Geometry: final body of the model. Coordinates: model frame, mm. A direction names the side the tool comes from. Round coordinates to 2 decimals unless told otherwise and drop trailing zeros. Write each loop counter-clockwise with the first axis right and the second up, starting at its lowest first coordinate (ties: lowest second). Pieces come first, ordered by that corner, then holes. Notation, with made-up numbers: M 86.25,74 L 110.25,74 A27 ccw 110.25,95 Z; hole C 79.25,18.25 d10. An arc over 180 degrees is marked long. Answer as CSV lines item,"result". Start each with the question number.
Q1. Section query A-A on y = 112.5. Output: boundary loops of the cut face in (x, z).
Q2. Section query C-C on x = 33. Output: boundary loops of the cut face in (y, z), and give its area (3 significant figures).
Q3. Section query B-B on z = 12.5. Output: boundary loops of the cut face in (x, y) (3 decimals), and give its area (3 significant figures).
Q4. First-contact query: pin 1 (4 mm diameter, centred on x = 86.5, y = 33, fed in from -Z); pin 2 (6 mm diameter, centred on y = 212.775, z = 4.5, fed in from +X); pin 3 (4.5 mm diameter, centred on x = 85, y = 132.5, fed in from -Z). Flat tips, straight axial feed; report the tip coordinate or a pass-through.
Q5. Ray query, probe 1 along X at (y, z) = (42.5, 14.5); probe 2 along X at (y, z) = (77.5, 14.25); probe 3 along Y at (x, z) = (-73.75, 4.5) (3 decimals). Return the intervals inside material, ascending.
Q6. Reachability of faces 4 (the flat face through (-87.9, 34.3, 2.1)), 5 (the flat face through (82, 137.775, 10)), 6 (the flat face through (-61.6, 30.1, 4.9)) from +Z, -Z, +X, -X, +Y, -Y: full face, straight path, thin tool, end or side. Return the list, or none.
Q7. Mould query, pull axis X, two halves, no side actions, for faces 1 (the flat face through (-81.5, 112, 15)), 2 (the flat face through (-82.5, 214, 7)), 3 (the flat face through (87, 133, 9)). Classes: pulls with the +X half, pulls with the -X half, needs draft (parallel to the pull), parting line crosses it, or undercut.
Q8. Section query D-D on y = 181.5. Output: boundary loops of the cut face in (x, z).
```python
from build123d import *

# Parameters (mm, degrees)
BOSS_EXTRUDE1_DEPTH = 10
BOSS_EXTRUDE2_DEPTH = 10
SKETCH3_W           = 9
SKETCH3_H           = 9
CUT_EXTRUDE2_DEPTH  = 10
SKETCH5_W           = 9
SKETCH5_H           = 9
CUT_EXTRUDE3_DEPTH  = 10
SKETCH6_R           = 2.25
CUT_EXTRUDE4_DEPTH  = 11
SKETCH7_R           = 2.25
CUT_EXTRUDE5_DEPTH  = 11
SKETCH8_R           = 1.75
CUT_EXTRUDE6_DEPTH  = 238.06159669
SKETCH9_R           = 1.75
CUT_EXTRUDE7_DEPTH  = 6
CHAMFER1_SIZE       = 0.5
CHAMFER1_SIZE2      = 1.866025404
CUT_EXTRUDE8_DEPTH  = 2.1


with BuildPart() as part:
    # Sketch1 → Boss-Extrude1 (new body)
    with BuildSketch(Plane.XY):
        Polygon((0, 0), (-91.5, 0), (-91.5, 217.775), (-71.5, 217.775), (-71.5, 40), (-51.5, 20), (0, 20), (51.5, 20), (71.5, 40), (71.5, 137.775), (91.5, 137.775), (91.5, 0), align=None)
    extrude(amount=BOSS_EXTRUDE1_DEPTH)

    # Sketch2 → Boss-Extrude2 (add)
    with BuildSketch(Plane.XY.offset(10)):
        Polygon((-81.5, 217.775), (-91.5, 217.775), (-91.5, 0), (91.5, 0), (91.5, 137.775), (81.5, 137.775), (81.5, 10), (-81.5, 10), align=None)
    extrude(amount=BOSS_EXTRUDE2_DEPTH)

    # Sketch3 → Cut-Extrude2 (cut)
    with BuildSketch(Plane(origin=(0, 217.775, 0), x_dir=(1, 0, 0), z_dir=(0, 1, 0))):
        with Locations((-87, -4.5)):
            Rectangle(SKETCH3_W, SKETCH3_H)
    extrude(amount=-CUT_EXTRUDE2_DEPTH, mode=Mode.SUBTRACT)

    # Sketch5 → Cut-Extrude3 (cut)
    with BuildSketch(Plane(origin=(0, 137.775, 0), x_dir=(1, 0, 0), z_dir=(0, 1, 0))):
        with Locations((87, -4.5)):
            Rectangle(SKETCH5_W, SKETCH5_H)
    extrude(amount=-CUT_EXTRUDE3_DEPTH, mode=Mode.SUBTRACT)

    # Sketch6 → Cut-Extrude4 (cut)
    with BuildSketch(Plane.ZY.offset(82.5)):
        with Locations((4.5, 212.775)):
            Circle(SKETCH6_R)
    extrude(amount=-CUT_EXTRUDE4_DEPTH, mode=Mode.SUBTRACT)

    # Sketch7 → Cut-Extrude5 (cut)
    with BuildSketch(Plane(origin=(82.5, 0, 0), x_dir=(0, 0, -1), z_dir=(1, 0, 0))):
        with Locations((-4.5, 132.775)):
            Circle(SKETCH7_R)
    extrude(amount=-CUT_EXTRUDE5_DEPTH, mode=Mode.SUBTRACT)

    # Sketch8 → Cut-Extrude6 (cut, through all)
    with BuildSketch(Plane(origin=(0, 0, 0), x_dir=(-1, 0, 0), z_dir=(0, 0, -1))):
        with Locations((86.5, 33)):
            Circle(SKETCH8_R)
        with Locations((-86.5, 33)):
            Circle(SKETCH8_R)
        with Locations((-86.5, 43)):
            Circle(SKETCH8_R)
        with Locations((86.5, 43)):
            Circle(SKETCH8_R)
    extrude(amount=-CUT_EXTRUDE6_DEPTH, mode=Mode.SUBTRACT)

    # Sketch9 → Cut-Extrude7 (cut)
    with BuildSketch(Plane(origin=(0, 20, 0), x_dir=(1, 0, 0), z_dir=(0, 1, 0))):
        with Locations(Location((-11, -5, 0), (0, 0, 270))):
            Circle(SKETCH9_R)
    extrude(amount=-CUT_EXTRUDE7_DEPTH, mode=Mode.SUBTRACT)

    # Chamfer1
    chamfer1_edges = [part.edges().sort_by_distance(p)[0] for p in [
        (-11, 20, 3.25),
    ]]
    chamfer1_side = [part.faces().sort_by_distance(p)[0] for p in [
        (0.103718732, 20, 5),
    ]]
    chamfer(chamfer1_edges, length=CHAMFER1_SIZE, length2=CHAMFER1_SIZE2, reference=chamfer1_side[0])

    # Sketch10 → Cut-Extrude8 (cut)
    with BuildSketch(Plane(origin=(0, 0, 0), x_dir=(-1, 0, 0), z_dir=(0, 0, -1))):
        Polygon((-84.854551733, 30.15), (-83.209103466, 33), (-84.854551733, 35.85), (-88.145448267, 35.85), (-89.790896534, 33), (-88.145448267, 30.15), align=None)
        Polygon((88.145448267, 30.15), (89.790896534, 33), (88.145448267, 35.85), (84.854551733, 35.85), (83.209103466, 33), (84.854551733, 30.15), align=None)
        Polygon((-84.854551733, 40.15), (-83.209103466, 43), (-84.854551733, 45.85), (-88.145448267, 45.85), (-89.790896534, 43), (-88.145448267, 40.15), align=None)
        Polygon((88.145448267, 40.15), (89.790896534, 43), (88.145448267, 45.85), (84.854551733, 45.85), (83.209103466, 43), (84.854551733, 40.15), align=None)
    extrude(amount=-CUT_EXTRUDE8_DEPTH, mode=Mode.SUBTRACT)


solid = part.part
```
Entries:
1,outline,"M -91.5,0 L -71.5,0 L -71.5,10 L -81.5,10 L -81.5,20 L -91.5,20 Z; M 71.5,0 L 91.5,0 L 91.5,20 L 81.5,20 L 81.5,10 L 71.5,10 Z"
2,outline,"M 0,0 L 20,0 L 20,10 L 10,10 L 10,20 L 0,20 Z"
2,area,"300 mm^2"
3,outline,"M -91.5,0 L 91.5,0 L 91.5,137.775 L 81.5,137.775 L 81.5,10 L -81.5,10 L -81.5,217.775 L -91.5,217.775 Z; hole C -86.5,33 d3.5; hole C -86.5,43 d3.5; hole C 86.5,33 d3.5; hole C 86.5,43 d3.5"
3,area,"5,150 mm^2"
4,pin 1,"stops at z = 2.1"
4,pin 2,"stops at x = -71.5"
4,pin 3,"stops at z = 9"
5,probe 1,"x = -91.5 to -88.18, -84.82 to -81.5, 81.5 to 84.82, 88.18 to 91.5"
5,probe 2,"x = -91.5 to -81.5, 81.5 to 91.5"
5,probe 3,"y = 0 to 210.525, 215.025 to 217.775"
6,face 4,"-Z"
6,face 5,"+Z, -Z, +X, +Y"
6,face 6,"+Z, -Z, +Y"
7,face 1,"undercut"
7,face 2,"pulls with the -X half"
7,face 3,"needs draft"
8,outline,"M -91.5,0 L -71.5,0 L -71.5,10 L -81.5,10 L -81.5,20 L -91.5,20 Z"
